For this review, use the dimensioned drawing (mm, ordinates from the lowest corner) and the shaded views. A direction names the side the tool comes from. Round coordinates to 2 decimals unless told otherwise and drop trailing zeros. Write each loop counter-clockwise with the first axis right and the second up, starting at its lowest first coordinate (ties: lowest second). Pieces come first, ordered by that corner, then holes. Notation, with made-up numbers: (17.25, 49) -> (54.25, 49) arc R25 cw to (54.25, 88) -> close; hole circle Ø3 at (-32.75, 46). An arc over 180 degrees is marked (long way). Write each question's results on one line, items separated by ' | '. Start each with the question number.
Item 1: The part is to be moulded in two halves that separate along Y. For the marked faces 1, 2 and 3, say which applies: +Y half, -Y half, draft (parallel to the pull), parting line (faces both ways), or undercut.
Item 2: Add section D-D (y = 71). Count the separate pieces of the cut face and the enclosed holes in it, plus the area to 3 significant figures.
Item 3: Add section B-B (z = 38.3). State the section outline as (x, y) points.
Item 4: Tool access review of the marked faces 4 and 5: name each direction out of +Z, -Z, +X, -X, +Y, -Y from which nothing blocks a thin tool from reaching the whole face with its end or side.
Item 5: Add section C-C (x = 20). State the section outline as (y, z) points.
Item 6: Add section A-A (y = 38.3). State the section outline as (x, z) points, plus the area to 3 significant figures.
Item 7: Clearance check with flat-ended pins moving along their axes: pin 1 (2 mm diameter, centred on x = 16.5, z = 23, fed in from +Y); pin 2 (12 mm diameter, centred on x = 14.5, z = 55, fed in from -Y); pin 3 (3 mm diameter, centred on x = 8, y = 15, fed in from +Z); pin 4 (17 mm diameter, centred on y = 38.3, z = 38.3, fed in from +X). State where each tip first meets the part, or that it passes through.
Item 8: To check wall thickness, follow line 1 along X through (y, z) = (67, 21.5); line 2 along X through (y, z) = (66, 40.5); line 3 along Z through (x, y) = (11.5, 38). State the ranges of each line that lie inside material, in increasing order.
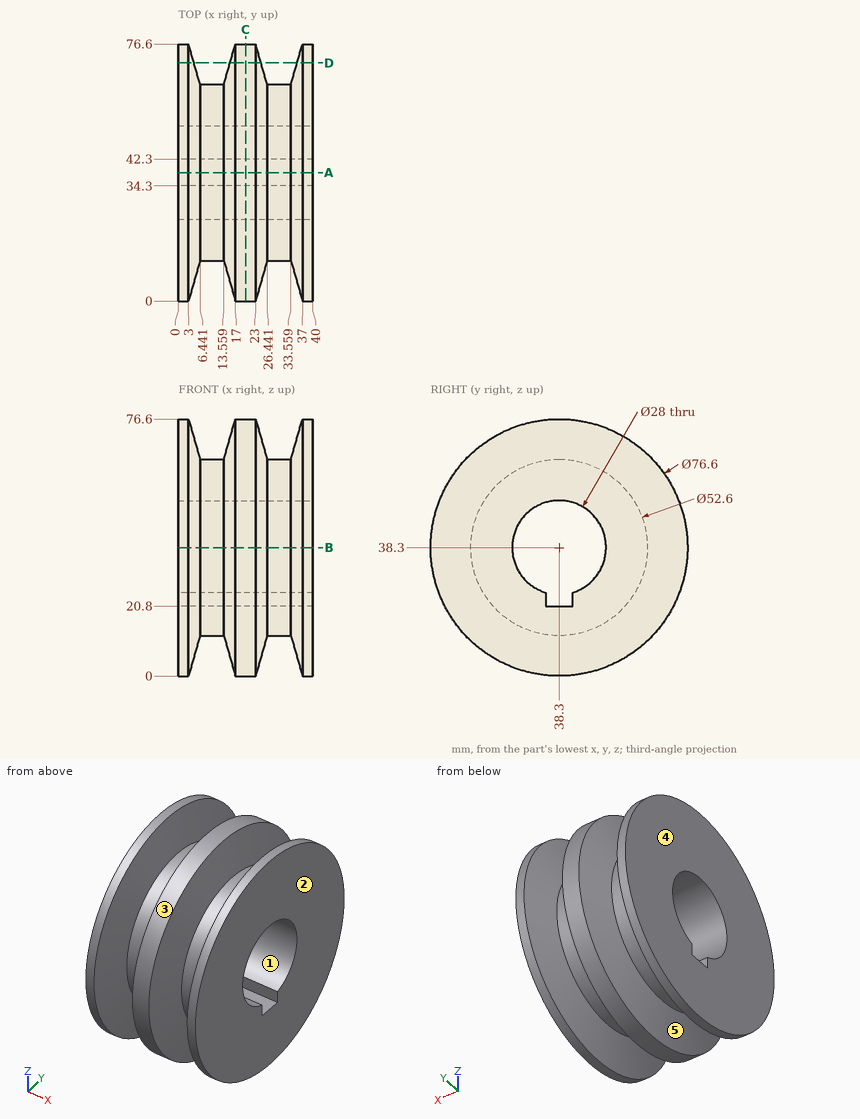
Responses:
1) face 1: undercut | face 2: draft | face 3: parting line
2) separate pieces: 3 | enclosed holes: 0 | area: 647 mm^2
3) outline: (0, 0) -> (3, 0) -> (6.44, 12) -> (13.56, 12) -> (17, 0) -> (23, 0) -> (26.44, 12) -> (33.56, 12) -> (37, 0) -> (40, 0) -> (40, 24.3) -> (0, 24.3) -> close; (0, 52.3) -> (40, 52.3) -> (40, 76.6) -> (37, 76.6) -> (33.56, 64.6) -> (26.44, 64.6) -> (23, 76.6) -> (17, 76.6) -> (13.56, 64.6) -> (6.44, 64.6) -> (3, 76.6) -> (0, 76.6) -> close
4) face 4: +Z, -Z, -X, +Y, -Y | face 5: none
5) outline: circle Ø76.6 at (38.3, 38.3); hole (34.3, 20.8) -> (42.3, 20.8) -> (42.3, 24.88) arc R14 ccw (long way) to (34.3, 24.88) -> close
6) outline: (0, 0) -> (3, 0) -> (6.44, 12) -> (13.56, 12) -> (17, 0) -> (23, 0) -> (26.44, 12) -> (33.56, 12) -> (37, 0) -> (40, 0) -> (40, 20.8) -> (0, 20.8) -> close; (0, 52.3) -> (40, 52.3) -> (40, 76.6) -> (37, 76.6) -> (33.56, 64.6) -> (26.44, 64.6) -> (23, 76.6) -> (17, 76.6) -> (13.56, 64.6) -> (6.44, 64.6) -> (3, 76.6) -> (0, 76.6) -> close | area: 1,300 mm^2
7) pin 1: stops at y = 73.78 | pin 2: stops at y = 1.69 | pin 3: stops at z = 53.01 | pin 4: passes through
8) line 1: x = 0 to 4.45, 15.55 to 24.45, 35.55 to 40 | line 2: x = 0 to 6.01, 13.99 to 26.01, 33.99 to 40 | line 3: z = 12 to 20.8, 52.3 to 64.6
